Answer from the drawing. Dimensions are ordinates in mm from the lowest x, y and z of the part. Round coordinates to 2 decimals unless told otherwise and drop trailing zeros. Write each loop counter-clockwise with the first axis right and the second up, starting at its lowest first coordinate (ties: lowest second). Pieces come first, ordered by that corner, then holes. Notation, with made-up numbers: (83, -33) -> (141, -33) arc R18 ccw to (141, -25) -> close; hole circle Ø8 at (82, 57). An arc over 180 degrees is marked (long way). Answer as a JSON object with one key per item and string values. Group by question number.
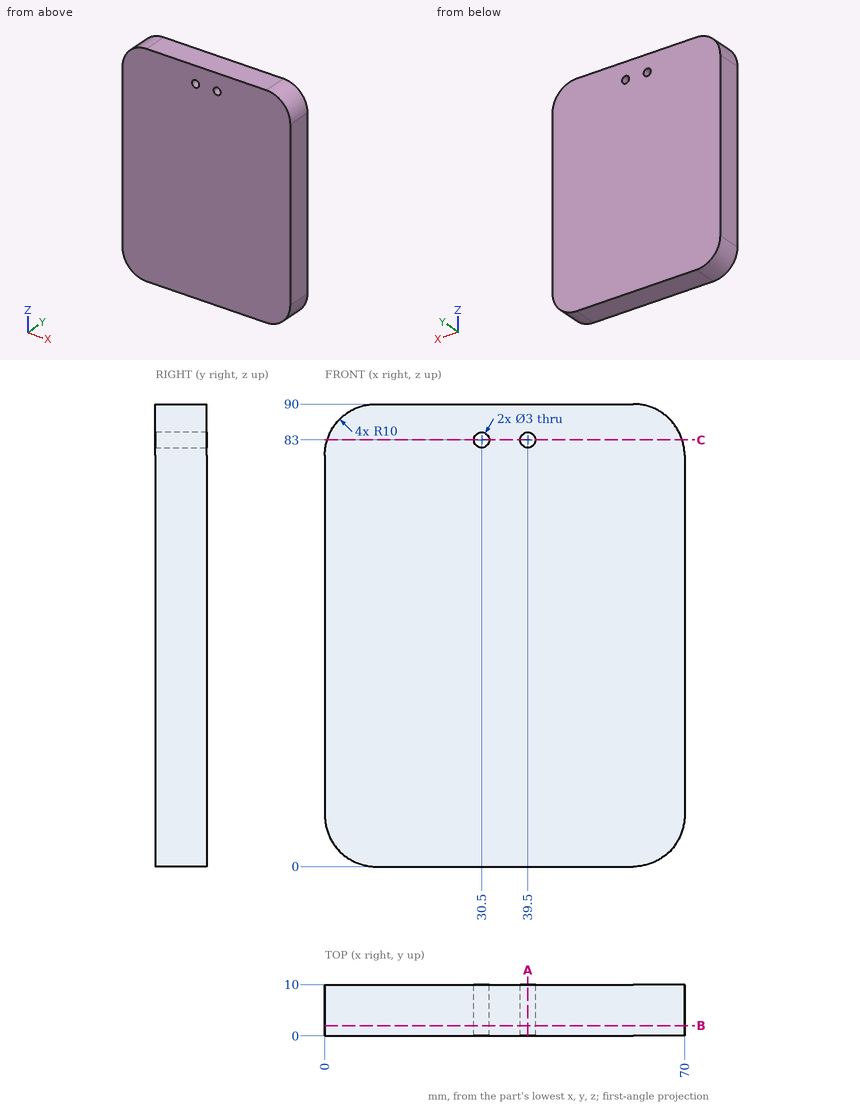
1) Straight lines are drawn through the part: L1, parallel to X at y = 7, z = 83; L2, parallel to Z at x = 30, y = 5.25; L3, parallel to X at y = 2.75, z = 82. For each, find the intervals that lie inside material, in ascending order.
2) A cutting plane is placed at A-A on x = 39.5. Determine the outline of the cut face in (y, z).
3) A cutting plane is placed at C-C on z = 83. Determine the outline of the cut face in (x, y), plus the area to 3 significant figures.
4) This flat-tipped pin is pushed along its axis until it touches: P1, Ø1.8, axis at x = 30.5, z = 83, coming from the +Y side. Where does it stop, or does it pass through?
5) A cutting plane is placed at B-B on y = 2. Determine the outline of the cut face in (x, z), plus the area to 3 significant figures.
Established:
{
 "1": {"L1": "x = 0.46 to 29, 32 to 38, 41 to 69.54", "L2": "z = 0 to 81.59, 84.41 to 90", "L3": "x = 0.2 to 29.38, 31.62 to 38.38, 40.62 to 69.8"},
 "2": {"outline": "(0, 0) -> (10, 0) -> (10, 81.5) -> (0, 81.5) -> close; (0, 84.5) -> (10, 84.5) -> (10, 90) -> (0, 90) -> close"},
 "3": {"outline": "(0.46, 0) -> (29, 0) -> (29, 10) -> (0.46, 10) -> close; (32, 0) -> (38, 0) -> (38, 10) -> (32, 10) -> close; (41, 0) -> (69.54, 0) -> (69.54, 10) -> (41, 10) -> close", "area": "631 mm²"},
 "4": {"P1": "passes through"},
 "5": {"outline": "(0, 10) arc R10 ccw to (10, 0) -> (60, 0) arc R10 ccw to (70, 10) -> (70, 80) arc R10 ccw to (60, 90) -> (10, 90) arc R10 ccw to (0, 80) -> close; hole circle Ø3 at (30.5, 83); hole circle Ø3 at (39.5, 83)", "area": "6,200 mm²"}
}
